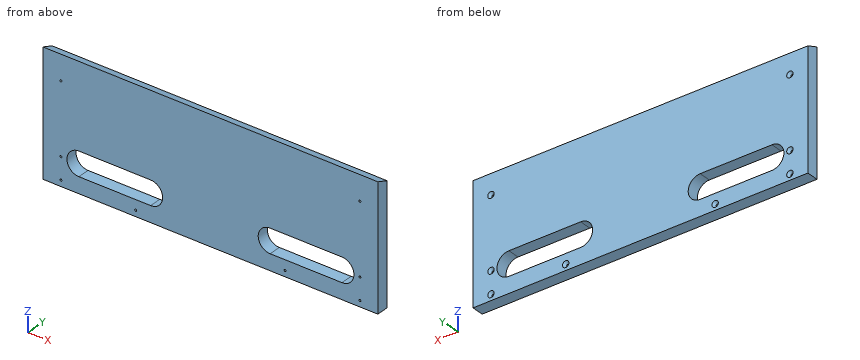
```python
from build123d import *

# Parameters (mm, degrees)
SKETCH1_W           = 533.146
SKETCH1_H           = 196.863399688
BOSS_EXTRUDE1_DEPTH = 19.05
CUT_EXTRUDE1_DEPTH  = 7702.120410186
CUT_EXTRUDE2_DEPTH  = 7008.877833132
HOLE1_D             = 3.175
HOLE1_DEPTH         = 38.1
HOLE1_CSINK_D       = 10.16
HOLE1_CSINK_ANGLE   = 82
HOLE1_TIP           = 0.953866233


with BuildPart() as part:
    # Sketch1 → Boss-Extrude1 (new body)
    with BuildSketch(Plane(origin=(0, 3140.71, 0), x_dir=(1, 0, 0), z_dir=(0, 1, 0))):
        with Locations((0, 6904.348295077)):
            Rectangle(SKETCH1_W, SKETCH1_H)
    extrude(amount=BOSS_EXTRUDE1_DEPTH)

    # Sketch2 → Cut-Extrude1 (cut, through all)
    with BuildSketch(Plane(origin=(266.573, 0, 0), x_dir=(0, 0, -1), z_dir=(1, 0, 0))):
        Polygon((6805.916595233, 3140.710000001), (6813.613294835, 3159.760000001), (6805.916595233, 3159.760000001), align=None)
    extrude(amount=-CUT_EXTRUDE1_DEPTH, mode=Mode.SUBTRACT)

    # Sketch3 → Cut-Extrude2 (cut, through all)
    with BuildSketch(Plane(origin=(0, 3159.76, 0), x_dir=(1, 0, 0), z_dir=(0, 1, 0))):
        with BuildLine():
            Line((209.423, 6939.279994921), (95.123, 6939.279994921))
            ThreePointArc((95.123, 6939.279994921), (76.073, 6958.329994921), (95.123, 6977.379994921))
            Line((95.123, 6977.379994921), (209.423, 6977.379994921))
            ThreePointArc((209.423, 6977.379994921), (228.473, 6958.329994921), (209.423, 6939.279994921))
        make_face()
        with BuildLine():
            Line((-209.423, 6939.279994921), (-95.123, 6939.279994921))
            ThreePointArc((-95.123, 6939.279994921), (-76.073, 6958.329994921), (-95.123, 6977.379994921))
            Line((-95.123, 6977.379994921), (-209.423, 6977.379994921))
            ThreePointArc((-209.423, 6977.379994921), (-228.473, 6958.329994921), (-209.423, 6939.279994921))
        make_face()
    extrude(amount=-CUT_EXTRUDE2_DEPTH, mode=Mode.SUBTRACT)

    # Hole1
    with Locations(Plane(origin=(0, 3159.76, 0), x_dir=(1, 0, 0), z_dir=(0, 1, 0))):
        with Locations((-118.999, 6993.254994921), (237.998, 6993.254994921), (237.998, 6958.329994921), (237.998, 6845.512682081), (-237.998, 6993.254994921), (-237.998, 6958.329994921), (-237.998, 6845.512682081), (118.999, 6993.254994921)):
            CounterSinkHole(HOLE1_D / 2, HOLE1_CSINK_D / 2, depth=HOLE1_DEPTH, counter_sink_angle=HOLE1_CSINK_ANGLE)
            with Locations((0, 0, -(HOLE1_DEPTH + HOLE1_TIP / 2))):  # 118° drill point
                Cone(0, HOLE1_D / 2, HOLE1_TIP, mode=Mode.SUBTRACT)


solid = part.part
```
Check sheet for the modelled part. Datum: model origin and axes. Units: mm. Round coordinates to 2 decimals unless told otherwise and drop trailing zeros. Order: outer loops, then holes, each group sorted by start corner. A loop starts at its lowest first (then second) coordinate and runs counter-clockwise, first axis right, second up. Notation, with made-up numbers: (-12, 20.5) -> (0, 20.5) arc R8 ccw to (0, 35.5) -> close; hole circle Ø5 at (46.25, 53). An arc over 180 degrees is marked (long way). One line per item, written item: value. Start each with the question number.
Q1. Gauge pin test, flat ends, axial feed: pin 1 Ø4 at (x, z) = (238, -6958.33) entering from +Y; pin 2 Ø3.5 at (x, z) = (-238, -6958.33) entering from +Y; pin 3 Ø9.5 at (x, y) = (176, 3152) entering from +Z. Record the tip position at first contact, or that the pin passes through.
Q2. Cross-section at C-C (y = 3150.75). Give the number of separate pieces and of enclosed holes in the cut face, and give its area (3 significant figures).
Q3. Cross-section at B-B (z = -6946.5). Record the boundary of the cut face in (x, y), and give its area (3 significant figures).
Q4. Cross-section at D-D (x = -4). Record the boundary of the cut face in (y, z), and give its area (3 significant figures).
Q5. Thickness scan on line 1 (X direction, y = 3148.25, z = -6944); line 2 (X direction, y = 3150.5, z = -6954); line 3 (Z direction, x = 184.5, y = 3149.75). Record the ranges inside material, lowest first.
Q6. Cross-section at A-A (x = 147.5). Record the boundary of the cut face in (y, z).
Completed:
1. pin 1: stops at y = 3156.22
1. pin 2: stops at y = 3155.93
1. pin 3: stops at z = -6808.56
2. separate pieces: 1
2. enclosed holes: 10
2. area: 91,700 mm²
3. outline: (-266.57, 3140.71) -> (-224.35, 3140.71) -> (-224.35, 3159.76) -> (-266.57, 3159.76) -> close; (-80.19, 3140.71) -> (80.19, 3140.71) -> (80.19, 3159.76) -> (-80.19, 3159.76) -> close; (224.35, 3140.71) -> (266.57, 3140.71) -> (266.57, 3159.76) -> (224.35, 3159.76) -> close
3. area: 4,660 mm²
4. outline: (3140.71, -7002.78) -> (3159.76, -7002.78) -> (3159.76, -6813.61) -> (3140.71, -6805.92) -> close
4. area: 3,680 mm²
5. line 1: x = -266.57 to -221.98, -82.57 to 82.57, 221.98 to 266.57
5. line 2: x = -266.57 to -227.97, -76.57 to 76.57, 227.97 to 266.57
5. line 3: z = -7002.78 to -6977.38, -6939.28 to -6809.57
6. outline: (3140.71, -7002.78) -> (3159.76, -7002.78) -> (3159.76, -6977.38) -> (3140.71, -6977.38) -> close; (3140.71, -6939.28) -> (3159.76, -6939.28) -> (3159.76, -6813.61) -> (3140.71, -6805.92) -> close
